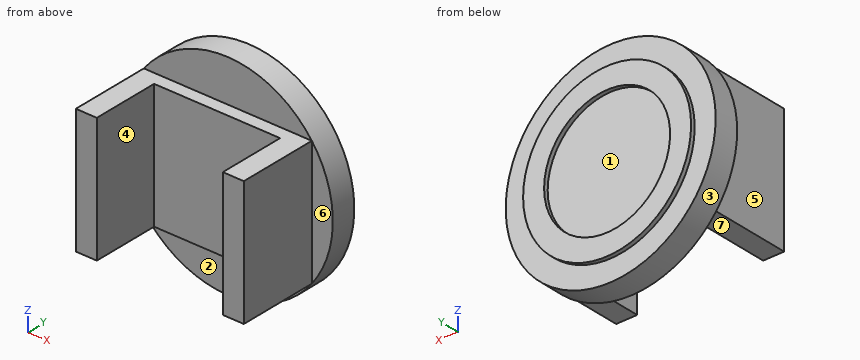
Autodesk Inventor part; units mm, degrees
ref_plane "Work Plane1" through (0, 50, 0) normal (0, 1, 0) x (-1, 0, 0)
sketch "Sketch1" plane through (0, 50, 0) normal (0, 1, 0) x (-1, 0, 0)
  circle A0 centre (0, 0) radius 50
  dimension "d11" = 100
extrude "Extrusion1" add sketch "Sketch1" against normal blind 12
sketch "Sketch2" plane through (0, 0, 0) normal (0, 0, 1) x (1, 0, 0)
  line L0 (-40, 38) -> (40, 38)
  line L1 (-40, 50) -> (-40, 38)
  line L2 (-40, 38) -> (-40, 0)
  line L3 (-40, 0) -> (-30, 0)
  line L4 (-30, 0) -> (-30, 32)
  line L5 (-30, 32) -> (30, 32)
  line L6 (30, 32) -> (30, 0)
  line L7 (30, 0) -> (40, 0)
  line L8 (40, 50) -> (40, 38)
  line L9 (40, 0) -> (40, 38)
  point P0 (0, 0)
  dimension "d5" = 10
  dimension "d6" = 32
  dimension "d7" = 60
  dimension "d8" = 10
extrude "Extrusion2" add sketch "Sketch2" along normal mid plane 60
sketch "Sketch3" plane through (0, 50, 0) normal (0, 1, 0) x (1, 0, 0)
  circle A0 centre (0, 0) radius 40
  circle A1 centre (0, 0) radius 30
  dimension "d12" = 80
  dimension "d15" = 60
extrude "Extrusion3" add sketch "Sketch3" along normal blind 2
properties part number "Z5" material "Steel, Alloy"
Verification items for the finished model (mm, model axes). Face numbers are marked on the shaded views. A direction names the side the tool comes from. Round coordinates to 2 decimals unless told otherwise and drop trailing zeros. Order: outer loops, then holes, each group sorted by start corner. A loop starts at its lowest first (then second) coordinate and runs counter-clockwise, first axis right, second up. Notation, with made-up numbers: (81, 65) - (121, 65) arc R20 ccw to (121, 83) - close; hole circle Ø4 at (63, 16.25). An arc over 180 degrees is marked (long way). Use CSV: the item, a comma, the result in double quotes. Start each with the question number.
1) Section check B-B, the plane z = 0. Record the cut outline in (x, y), plus the area to 3 significant figures.
2) Section check A-A, the plane y = 21. Record the cut outline in (x, z), plus the area to 3 significant figures.
3) Mould release check, pull along X, two halves, no side actions. Record for the marked faces 1, 2, 3 and 4: +X half, -X half, draft (parallel to the pull), parting line (faces both ways), or undercut.
4) Access from +Z, -Z, +X, -X, +Y, -Y to the whole of each face (thin tool, end or side, straight path). Record for the marked faces 5, 6 and 7.
5) Thickness scan on L1, parallel to X at y = 11.5, z = -20.5; L2, parallel to Y at x = -21, z = -32. Record the ranges inside material, lowest first.
6) Section check C-C, the plane x = 0. Record the cut outline in (y, z).
7) Go/stop test with flat-tipped pins: P1, Ø9.5, axis at y = 15.5, z = 0.5, coming from the -X side; P2, Ø9.5, axis at y = 14.5, z = 1, coming from the +X side; P3, Ø3, axis at x = 46, z = 5, coming from the -Y side; P4, Ø8, axis at x = 1, y = 26, coming from the +Z side. Record where each tip stops, or that it passes through.
8) Section check D-D, the plane y = 46. Record the cut outline in (x, z).
Answers:
1,outline,"(-50, 38) - (-40, 38) - (-40, 0) - (-30, 0) - (-30, 32) - (30, 32) - (30, 0) - (40, 0) - (40, 38) - (50, 38) - (50, 50) - (40, 50) - (40, 52) - (30, 52) - (30, 50) - (-30, 50) - (-30, 52) - (-40, 52) - (-40, 50) - (-50, 50) - close"
1,area,"2,360 mm²"
2,outline,"(-40, -30) - (-30, -30) - (-30, 30) - (-40, 30) - close; (30, -30) - (40, -30) - (40, 30) - (30, 30) - close"
2,area,"1,200 mm²"
3,face 1,"undercut"
3,face 2,"draft"
3,face 3,"parting line"
3,face 4,"undercut"
4,face 5,"+Z, -Z, -X, -Y"
4,face 6,"+Z, -Z, +X, -Y"
4,face 7,"-Z, +X, -X, -Y"
5,L1,"x = -40 to -30, 30 to 40"
5,L2,"y = 38 to 52"
6,outline,"(32, -30) - (38, -30) - (38, -50) - (50, -50) - (50, -40) - (52, -40) - (52, -30) - (50, -30) - (50, 30) - (52, 30) - (52, 40) - (50, 40) - (50, 50) - (38, 50) - (38, 30) - (32, 30) - close"
7,P1,"stops at x = -40"
7,P2,"stops at x = 40"
7,P3,"stops at y = 38"
7,P4,"passes through"
8,outline,"circle Ø100 at (0, 0)"
